Geometry: final body of the model. Coordinates: model frame, mm. Give positions to 0.01 mm unless a question says otherwise; leave off trailing zeros. Loops run counter-clockwise (first coordinate to the right, second up) from the corner with the lowest first, then second, coordinate; pieces in that order, holes last.
1. Material intervals for line 1 along Y through (x, z) = (27.5, 0.6); line 2 along X through (y, z) = (-26, 0.55); line 3 along Y through (x, z) = (-31.5, 1.75), sorted ascending.
2. First-contact query: P1, Ø1.5, axis at x = 22, y = 25.5, coming from the -Z side. Flat tip, straight axial feed; report the tip coordinate or a pass-through.
3. Section A-A, the plane y = -30. Output: boundary loops of the cut face in (x, z).
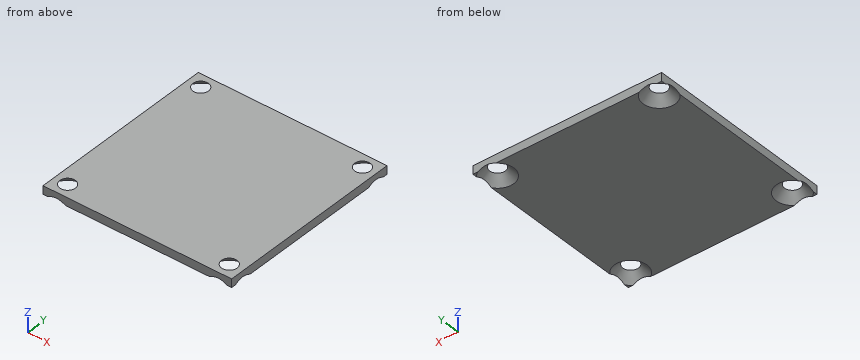
from build123d import *

# Parameters (mm, degrees)
F0_W           = 70
F0_H           = 70
F0_W_2         = 60
F0_H_2         = 60
F1_DEPTH       = 3.1
F2_D           = 4
F2_DEPTH       = 15
F2_CSINK_D     = 12
F2_CSINK_ANGLE = 90
F2_TIP         = 1.2017212381


with BuildPart() as f1:
    # F0 (on Top) → F1 (new body)
    with BuildSketch(Plane.XY):
        Rectangle(F0_W, F0_H)
        Rectangle(F0_W_2, F0_H_2, mode=Mode.SUBTRACT)
        Rectangle(F0_W_2, F0_H_2)
    extrude(amount=F1_DEPTH)

    # F2
    with Locations(Plane(origin=(0, 0, 0), x_dir=(1, 0, 0), z_dir=(0, 0, -1))):
        with Locations((-30, -30), (30, -30), (30, 30), (-30, 30)):
            CounterSinkHole(F2_D / 2, F2_CSINK_D / 2, depth=F2_DEPTH, counter_sink_angle=F2_CSINK_ANGLE)
            with Locations((0, 0, -(F2_DEPTH + F2_TIP / 2))):  # 118° drill point
                Cone(0, F2_D / 2, F2_TIP, mode=Mode.SUBTRACT)


solid = f1.part
Answers below:
1. line 1: y = -35 to -34.79, -25.21 to 25.21, 34.79 to 35
1. line 2: x = -35 to -33.7, -26.3 to 26.3, 33.7 to 35
1. line 3: y = -35 to -33.98, -26.02 to 26.02, 33.98 to 35
2. P1: stops at z = 0
3. outline: (-35, 1) - (-32.9, 3.1) - (-35, 3.1) - close; (-27.1, 3.1) - (-24, 0) - (24, 0) - (27.1, 3.1) - close; (32.9, 3.1) - (35, 1) - (35, 3.1) - close
